from build123d import *

# Parameters (mm, degrees)
BOX006_W               = 1168.4
BOX006_H               = 25.4
BOX006_DEPTH           = 1500
BOX005_W               = 1219.2
BOX005_H               = 609.6
BOX005_DEPTH           = 1500
CUT004_PLACEMENT_ANGLE = 270


with BuildPart() as cube006:
    # Box006 → Box006 (new body)
    with BuildSketch(Plane(origin=(25.4, 0, 25.4), x_dir=(1, 0, 0), z_dir=(0, 0, 1))):
        with Locations((584.2, 12.7)):
            Rectangle(BOX006_W, BOX006_H)
    extrude(amount=BOX006_DEPTH)


with BuildPart() as cut004:
    # Box005 → Box005 (new body)
    with BuildSketch(Plane.XY):
        with Locations((609.6, 304.8)):
            Rectangle(BOX005_W, BOX005_H)
    extrude(amount=BOX005_DEPTH)

    # Cut004: cut Cube006
    add(cube006.part, mode=Mode.SUBTRACT)


with BuildPart() as cut004_1:
    # Cut004 placement: moved
    add(cut004.part.moved(Location((4298, 2552, 0))).rotate(Axis((4298, 2552, 0), (0, 0, 1)), CUT004_PLACEMENT_ANGLE))


solid = cut004_1.part
Work out the finished part from the listing and answer in its coordinate system (mm). Give positions to 0.01 mm unless a question says otherwise; leave off trailing zeros. Order: outer loops, then holes, each group sorted by start corner. A loop starts at its lowest first (then second) coordinate and runs counter-clockwise, first axis right, second up. Notation, with made-up numbers: (32, -19) -> (39, -19) arc R18 ccw to (39, -13) -> close; hole circle Ø8 at (-2.75, 3.25). An arc over 180 degrees is marked (long way). Answer as a JSON object with one key per item and string values. Group by question number.
1. A flat-ended cylindrical pin translates along its axis: pin 1 Ø10 at (y, z) = (1606.5, 369) entering from -X. Find the tip coordinate at first contact, or state that the pin passes through.
2. Section B-B on y = 1644.5 is taken. Determine the outline of the cut face in (x, z), plus the area to 3 significant figures.
3. The mould has two halves that part along Y. Classify faces 1 (the flat face through (4323.4, 1951, 752)), 2 (the flat face through (4599, 2552, 740)), 3 (the flat face through (4599, 1332.8, 740)), 4 (the flat face through (4907.6, 1951, 740)): released by +Y, released by -Y, zero draft, split by the parting line, or undercut.
4. Consider line 1 along X through (y, z) = (2404, 1330.5). Determine where the line is inside the solid, lowest interval first. Write a range as [from, to].
5. Section A-A on z = 1023 is taken. Determine the outline of the cut face in (x, y).
Result sheet:
{
 "1": {"pin 1": "stops at x = 4323.4"},
 "2": {"outline": "(4298, 0) -> (4907.6, 0) -> (4907.6, 1500) -> (4323.4, 1500) -> (4323.4, 25.4) -> (4298, 25.4) -> close", "area": "877,000 mm^2"},
 "3": {"face 1": "undercut", "face 2": "released by +Y", "face 3": "released by -Y", "face 4": "zero draft"},
 "4": {"line 1": "x = [4323.4, 4907.6]"},
 "5": {"outline": "(4298, 1332.8) -> (4907.6, 1332.8) -> (4907.6, 2552) -> (4298, 2552) -> (4298, 2526.6) -> (4323.4, 2526.6) -> (4323.4, 1358.2) -> (4298, 1358.2) -> close"}
}
